Geometry: final body of the model. Coordinates: model frame, mm. Round coordinates to 2 decimals unless told otherwise and drop trailing zeros. Order: outer loops, then holes, each group sorted by start corner. A loop starts at its lowest first (then second) coordinate and runs counter-clockwise, first axis right, second up. Notation, with made-up numbers: M 5,16 L 55,16 A30 ccw 55,40 Z; hole C 71.25,35 d10. An arc over 180 degrees is marked long. Return JSON: item names as keys, results as strings. Group by question number.
Q1. Cut plane A-A on x = 0. Output: boundary loops of the cut face in (y, z).
Q2. Cut plane D-D on z = 3.9. Output: boundary loops of the cut face in (x, y), and give its area (3 significant figures).
Q3. Contact query for flat-ended pins moving along their axis: pin 1 (16 mm diameter, centred on x = 0, y = 0, fed in from +Z); pin 2 (10.5 mm diameter, centred on x = -20, y = 0, fed in from +Z). Output: stop coordinate, or through.
Q4. Cut plane C-C on x = 20. Output: boundary loops of the cut face in (y, z).
Q5. Cut plane B-B on z = 0.8. Output: boundary loops of the cut face in (x, y).
Q6. Ray query, probe 1 along Y at (x, z) = (0, 1.2); probe 2 along Y at (x, z) = (-20, 0.7); probe 3 along X at (y, z) = (3.5, 3.3). Return the intervals inside material, ascending.
Q7. Mould query, pull axis X, two halves, no side actions, for faces 1 (the face through (29, 0, 2)), 2 (the face through (6, 9, 0)), 3 (the face through (-1.172, 8.923, 2.465)). Classes: released by +X, released by -X, zero draft, split by the parting line, or undercut.
```python
from build123d import *

# Parameters (mm, degrees)
ESQUISSE1_W                = 58
ESQUISSE1_H                = 39
ESQUISSE1_R                = 9
BOSS_EXTRU_1_DEPTH         = 5
R_P_TITION_LIN_AIRE1_COUNT = 2
R_P_TITION_LIN_AIRE1_PITCH = 40


with BuildPart() as part:
    # Esquisse1 → Boss.-Extru.1 (new body)
    with BuildSketch(Plane.XY):
        Rectangle(ESQUISSE1_W, ESQUISSE1_H)
        Circle(ESQUISSE1_R, mode=Mode.SUBTRACT)
    extrude(amount=BOSS_EXTRU_1_DEPTH)

    # Esquisse3 → Fraisage pour vis à tête fraisée à 6 pans creux M61 (revolve, cut)
    with BuildSketch(Plane(origin=(20, 0, 5), x_dir=(0, -1, 0), z_dir=(1, 0, 0))):
        Polygon((0, 0), (0, 5), (3.25, 5), (3.25, 3), (6.25, 0), align=None)
    fraisage_pour_vis_t_te_frais_e_6_pan = revolve(axis=Axis((20, 0, 11.35), (0, 0, -1)), mode=Mode.SUBTRACT)

    # Répétition linéaire1: Fraisage pour vis à tête fraisée à 6 pans creux M61 ×2
    with Locations(*[(-i * R_P_TITION_LIN_AIRE1_PITCH, 0, 0) for i in range(1, R_P_TITION_LIN_AIRE1_COUNT)]):
        add(fraisage_pour_vis_t_te_frais_e_6_pan, mode=Mode.SUBTRACT)


solid = part.part
```
Result sheet:
{
 "1": {"outline": "M -19.5,0 L -9,0 L -9,5 L -19.5,5 Z; M 9,0 L 19.5,0 L 19.5,5 L 9,5 Z"},
 "2": {"outline": "M -29,-19.5 L 29,-19.5 L 29,19.5 L -29,19.5 Z; hole C -20,0 d10.3; hole C 0,0 d18; hole C 20,0 d10.3", "area": "1,840 mm²"},
 "3": {"pin 1": "passes through", "pin 2": "stops at z = 4"},
 "4": {"outline": "M -19.5,0 L -3.25,0 L -3.25,2 L -6.25,5 L -19.5,5 Z; M 3.25,0 L 19.5,0 L 19.5,5 L 6.25,5 L 3.25,2 Z"},
 "5": {"outline": "M -29,-19.5 L 29,-19.5 L 29,19.5 L -29,19.5 Z; hole C -20,0 d6.5; hole C 0,0 d18; hole C 20,0 d6.5"},
 "6": {"probe 1": "y = -19.5 to -9, 9 to 19.5", "probe 2": "y = -19.5 to -3.25, 3.25 to 19.5", "probe 3": "x = -29 to -22.91, -17.09 to -8.29, 8.29 to 17.09, 22.91 to 29"},
 "7": {"face 1": "released by +X", "face 2": "zero draft", "face 3": "undercut"}
}
